```python
from build123d import *

# Parameters (mm, degrees)
F0_W   = 30
F0_H   = 110
F0_H_2 = 80
F0_H_3 = 48.918920987
F0_W_2 = 170
F2_R   = 40
F3_R   = 40
F4_R   = 70


with BuildPart() as f1:
    # F0 (on Top) → F1 (revolve)
    with BuildSketch(Plane.XY):
        Polygon((-30, 670), (0, 670), (0, 750), (-200, 750), (-200, 670), align=None)
        with Locations((-15, 615)):
            Rectangle(F0_W, F0_H)
        with Locations((-15, 520)):
            Rectangle(F0_W, F0_H_2)
        with Locations((-15, 455.5405395065)):
            Rectangle(F0_W, F0_H_3)
        with Locations((-115, 520)):
            Rectangle(F0_W_2, F0_H_2)
        Polygon((-50, 81.081079013), (0, 81.081079013), (0, 431.081079013), (-30, 431.081079013), (-50, 431.081079013), align=None)
        Polygon((-315, 81.081079013), (-315, 0), (0, 0), (0, 81.081079013), (-50, 81.081079013), align=None)
    revolve(axis=Axis((0, 590.3630256653, 0), (0, 1, 0)))

    # F2
    f2_edges = [f1.edges().sort_by_distance(p)[0] for p in [
        (200, 750, 0),
    ]]
    fillet(f2_edges, radius=F2_R)

    # F3
    f3_edges = [f1.edges().sort_by_distance(p)[0] for p in [
        (200, 560, 0),
    ]]
    fillet(f3_edges, radius=F3_R)

    # F4
    f4_edges = [f1.edges().sort_by_distance(p)[0] for p in [
        (315, 81.081079, 0),
    ]]
    fillet(f4_edges, radius=F4_R)


solid = f1.part
```
Check sheet for the modelled part. Datum: model origin and axes. Units: mm. A direction names the side the tool comes from. Coordinates: 2 decimals unless noted, no trailing zeros. Write each loop counter-clockwise with the first axis right and the second up, starting at its lowest first coordinate (ties: lowest second). Pieces come first, ordered by that corner, then holes. Notation, with made-up numbers: (-30.5, 81.5) -> (-20.5, 81.5) arc R31 ccw to (-20.5, 106.5) -> close; hole circle Ø8 at (67, 59.5). An arc over 180 degrees is marked (long way). Use a Markdown table: item, result.
1. Sectioned sample at D-D (z = 121). Give the number of separate pieces and of enclosed holes in the cut face, plus the area to 3 significant figures.
Reported:
| item | result |
|---|---|
| separate pieces | 3 |
| enclosed holes | 0 |
| area | 94,000 mm2 |
2. Tool access check on faces 5 (the cylindrical face through (68.29, 5.46, -307.51)), 6 (the cylindrical face through (-190.764, 500.28, 60.075)), 7 (the cylindrical face through (29.97, 614.23, 1.32)). Record the directions out of +Z, -Z, +X, -X, +Y, -Y that give a thin tool (end or side, any length) a straight path to the whole face; none if there is none.
Reported:
| item | result |
|---|---|
| face 5 | +Y, -Y |
| face 6 | +Y |
| face 7 | none |
3. Scan lines: line 1 along Y through (x, z) = (90, 31); line 2 along Y through (x, z) = (27.5, 18); line 3 along Y through (x, z) = (57, 228). Record each from-to range of solid material in increasing order.
Reported:
| item | result |
|---|---|
| line 1 | y = 0 to 81.08, 480 to 560, 670 to 750 |
| line 2 | y = 0 to 431.08, 480 to 560, 670 to 750 |
| line 3 | y = 0 to 81.08 |
4. Release check for a two-part mould opening along Y. For faces 1 (the flat face through (22, 431.081, -22)), 2 (the flat face through (-2, 750, 2)), 3 (the cylindrical face through (-190.764, 689.72, 60.075)), 4 (the cylindrical face through (-47.69, 253.63, 15.02)) record: pulls with the +Y half, pulls with the -Y half, needs draft (parallel to the pull), parting line crosses it, or undercut.
Reported:
| item | result |
|---|---|
| face 1 | undercut |
| face 2 | pulls with the +Y half |
| face 3 | needs draft |
| face 4 | undercut |
5. Sectioned sample at C-C (y = 467.5). Enter the section's corners in (x, z).
Reported:
| item | result |
|---|---|
| outline | circle Ø60 at (0, 0) |
6. Go/stop test with a flat-tipped pin: pin 1 Ø12 at (y, z) = (318, 36) entering from +X. Record where the tip stops, or that it passes through.
Reported:
| item | result |
|---|---|
| pin 1 | stops at x = 40 |
